Part print with two shaded views. Sizes in mm from the minimum x, y, z corner. A direction names the side the tool comes from. Coordinates: 2 decimals unless noted, no trailing zeros. Loops run counter-clockwise (first coordinate to the right, second up) from the corner with the lowest first, then second, coordinate; pieces in that order, holes last. Notation, with made-up numbers: M -11,2.25 L 11,2.25 A22 ccw 11,16.25 Z; hole C 23.25,16.5 d2. An arc over 180 degrees is marked long. Write item = value, one per line. Start each with the question number.
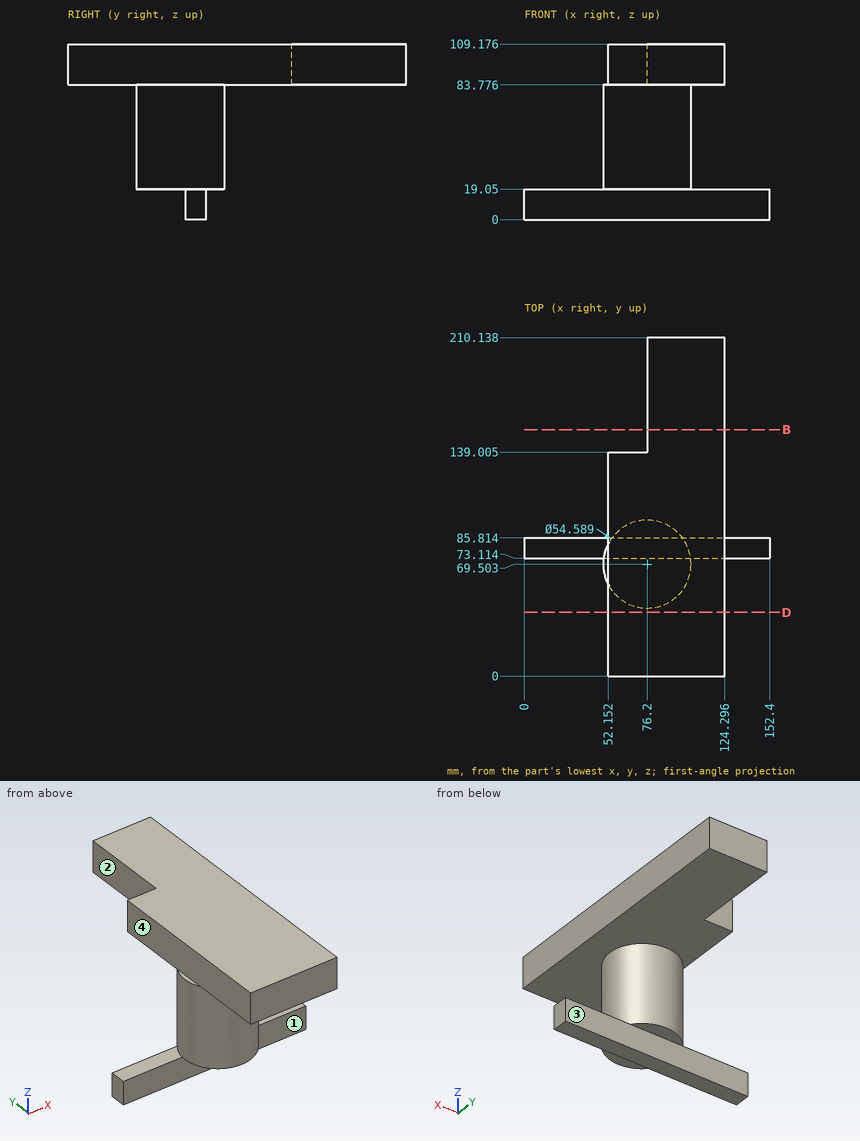
Item 1: Cut at B-B (y = 153). Give the cut face in (x, z) (1 decimal), plus the area to 3 significant figures.
Item 2: Pin check, flat tips, straight feed: pin 1 Ø12 at (y, z) = (106, 59) entering from -X; pin 2 Ø20.5 at (y, z) = (131, 93) entering from +X; pin 3 Ø12 at (y, z) = (125, 85) entering from -X; pin 4 Ø10 at (x, y) = (36.5, 81.5) entering from +Z. Stop position of each tip, or through.
Item 3: 3-axis set-ups, long thin cutter, end or side, ignore diameter. For the marked faces 1, 2, 3 and 4: which of +Z, -Z, +X, -X, +Y, -Y reach the whole face in a straight line?
Item 4: Cut at D-D (y = 39.5). Give the cut face in (x, z) (1 decimal), plus the area to 3 significant figures.
Item 5: Probe L1, parallel to Z at x = 116.5, y = 93.5; L2, parallel to Z at x = 83, y = 88.5; L3, parallel to X at y = 71.5, z = 22. List the from-to ranges inside material, lowest first.
Reported:
q1.outline = M 76.2,83.8 L 124.3,83.8 L 124.3,109.2 L 76.2,109.2 Z
q1.area = 1,220 mm^2
q2.pin_1 = through
q2.pin_2 = 124.3
q2.pin_3 = 52.15
q2.pin_4 = 19.05
q3.face_1 = -Z, +X, -X, -Y
q3.face_2 = +Z, -Z, -X, +Y
q3.face_3 = -Z, +X, -X, +Y
q3.face_4 = +Z, -X, +Y, -Y
q4.outline = M 52.2,83.8 L 124.3,83.8 L 124.3,109.2 L 52.2,109.2 Z
q4.area = 1,830 mm^2
q5.L1 = 83.78 to 109.18
q5.L2 = 19.05 to 109.18
q5.L3 = 48.98 to 103.42
